from build123d import *

# Parameters (mm, degrees)
ESQUISSE1_W             = 13.74
ESQUISSE1_H             = 13.74
BOSS_EXTRU_1_DEPTH      = 10.5
ESQUISSE3_R             = 4.4
ENL_V_MAT_EXTRU_2_DEPTH = 10
ESQUISSE8_R             = 5.5
BOSS_EXTRU_2_DEPTH      = 22
ESQUISSE2_R             = 2.8
ENL_V_MAT_EXTRU_3_DEPTH = 22
BOSS_EXTRU_3_DEPTH      = 22


with BuildPart() as part:
    # Esquisse1 → Boss.-Extru.1 (new body)
    with BuildSketch(Plane.XY):
        with Locations((-30.186071131, 8.6104)):
            Rectangle(ESQUISSE1_W, ESQUISSE1_H)
    extrude(amount=BOSS_EXTRU_1_DEPTH)

    # Esquisse3 → Enlèv. mat.-Extru.2 (cut)
    with BuildSketch(Plane.XY.offset(10.5)):
        with Locations((-30.186071131, 8.6104)):
            Circle(ESQUISSE3_R)
    extrude(amount=-ENL_V_MAT_EXTRU_2_DEPTH, mode=Mode.SUBTRACT)

    # Esquisse8 → Boss.-Extru.2 (add)
    with BuildSketch(Plane(origin=(0, 0, 0), x_dir=(-1, 0, 0), z_dir=(0, 0, -1))):
        with Locations(Location((30.186071131, 8.6104, 0), (0, 0, 180))):
            Circle(ESQUISSE8_R)
    extrude(amount=BOSS_EXTRU_2_DEPTH)

    # Esquisse2 → Enlèv. mat.-Extru.3 (cut)
    with BuildSketch(Plane(origin=(0, 0, 0), x_dir=(-1, 0, 0), z_dir=(0, 0, -1))):
        with Locations((30.186071131, 8.6104)):
            Circle(ESQUISSE2_R)
    extrude(amount=ENL_V_MAT_EXTRU_3_DEPTH, mode=Mode.SUBTRACT)

    # Esquisse9 → Boss.-Extru.3 (add)
    with BuildSketch(Plane(origin=(0, 0, -22), x_dir=(-1, 0, 0), z_dir=(0, 0, -1))):
        with BuildLine():
            Line((32.558926644, 10.096857773), (28.881418946, 11.087875061))
            ThreePointArc((28.881418946, 11.087875061), (30.919504526, 11.332054799), (32.558926644, 10.096857773))
        make_face()
    extrude(amount=-BOSS_EXTRU_3_DEPTH)


solid = part.part
Geometry: final body of the model. Coordinates: model frame, mm. A direction names the side the tool comes from. Give positions to 0.01 mm unless a question says otherwise; leave off trailing zeros. Write each loop counter-clockwise with the first axis right and the second up, starting at its lowest first coordinate (ties: lowest second). Pieces come first, ordered by that corner, then holes.
(1) Cut plane C-C, the plane z = 1.5. Return loops of the section in (x, y).
(2) Mould query, pull axis Y, two halves, no side actions, for faces 1 (the flat face through (-30, 15.48, 5)), 2 (the flat face through (-30.746, 10.585, -11.154)), 3 (the flat face through (-30, 1.74, 5)), 4 (the cylindrical face through (-27.82, 12.32, 5.57)). Classes: released by +Y, released by -Y, zero draft, split by the parting line, or undercut.
(3) Cut plane A-A, the plane x = -33.75. Return loops of the section in (y, z), then the cut area to 3 significant figures.
(4) Cut plane B-B, the plane y = 7. Return loops of the section in (x, z), then the cut area to 3 significant figures.
(5) First-contact query: P1, Ø8, axis at x = -30.19, y = 8.61, coming from the -Z side; P2, Ø5, axis at x = -30.19, y = 8.61, coming from the +Z side; P3, Ø1, axis at y = 3.5, z = -5, coming from the -X side; P4, Ø8, axis at y = 6.5, z = -13.5, coming from the -X side. Flat tips, straight axial feed; report the tip coordinate or a pass-through.
(6) Access query for faces 5 (the cylindrical face through (-29.37, 5.93, -10.85)), 6 (the flat face through (-37.056, 9, 5)), 7 (the flat face through (-30, 9, 0.5)). Directions: +Z, -Z, +X, -X, +Y, -Y. A direction counts if a zero-diameter tool reaches every point of the face in a straight line with its end or side. Return the directions, or none.
(7) Ray query, line 1 (X direction, y = 8.75, z = -11.5); line 2 (Y direction, x = -30.25, z = -19); line 3 (Y direction, x = -29.5, z = 4). Return the intervals inside material, ascending.
(8) Cut plane D-D, the plane x = -26.25. Return loops of the section in (y, z), then the cut area to 3 significant figures.
Values follow:
1. outline: (-37.06, 1.74) - (-23.32, 1.74) - (-23.32, 15.48) - (-37.06, 15.48) - close; hole circle Ø8.8 at (-30.19, 8.61)
2. face 1: released by +Y
2. face 2: undercut
2. face 3: released by -Y
2. face 4: undercut
3. outline: (1.74, 0) - (4.42, 0) - (4.42, -22) - (12.8, -22) - (12.8, 0) - (15.48, 0) - (15.48, 10.5) - (11.19, 10.5) - (11.19, 0.5) - (6.03, 0.5) - (6.03, 10.5) - (1.74, 10.5) - close
3. area: 277 mm2
4. outline: (-37.06, 0) - (-35.45, 0) - (-35.45, -22) - (-32.48, -22) - (-32.48, 0) - (-27.9, 0) - (-27.9, -22) - (-24.93, -22) - (-24.93, 0) - (-23.32, 0) - (-23.32, 10.5) - (-26.09, 10.5) - (-26.09, 0.5) - (-34.28, 0.5) - (-34.28, 10.5) - (-37.06, 10.5) - close
4. area: 193 mm2
5. P1: stops at z = -22
5. P2: stops at z = 0.5
5. P3: stops at x = -33.19
5. P4: stops at x = -35.69
6. face 5: -Z
6. face 6: +Z, -Z, -X, +Y, -Y
6. face 7: +Z
7. line 1: x = -35.68 to -32.98, -27.39 to -24.69
7. line 2: y = 3.11 to 5.81, 10.72 to 14.11
7. line 3: y = 1.74 to 4.26, 12.96 to 15.48
8. outline: (1.74, 0) - (4.77, 0) - (4.77, -22) - (12.45, -22) - (12.45, 0) - (15.48, 0) - (15.48, 10.5) - (10.58, 10.5) - (10.58, 0.5) - (6.64, 0.5) - (6.64, 10.5) - (1.74, 10.5) - close
8. area: 274 mm2
